Autodesk Inventor part; units mm, degrees
ref_plane "YZ Plane" through (0, 0, 0) normal (1, 0, 0) x (0, 1, 0)
ref_plane "XZ Plane" through (0, 0, 0) normal (0, 1, 0) x (-1, 0, 0)
ref_plane "XY Plane" through (0, 0, 0) normal (0, 0, 1) x (1, 0, 0)
sketch "Sketch1" plane through (0, 0, 0) normal (0, 0, 1) x (1, 0, 0)
  line L0 (-14.5, 28) -> (14.5, 28)
  line L1 (14.5, 28) -> (14.5, -28)
  line L2 (14.5, -28) -> (-14.5, -28)
  line L3 (-14.5, -28) -> (-14.5, 28)
  line L4 (17.5, 31) -> (-17.5, 31)
  line L5 (-17.5, 31) -> (-17.5, -31)
  line L6 (-17.5, -31) -> (17.5, -31)
  line L7 (14.5, -1.5) -> (26.5, -1.5)
  line L8 (14.5, -14.5) -> (26.5, -14.5)
  line L9 (17.5, -31) -> (17.5, -14.5)
  line L10 (17.5, -1.5) -> (17.5, 31)
  line L11 (26.5, -1.5) -> (26.5, -5)
  line L12 (26.5, -5) -> (14.5, -5)
  line L13 (26.5, -14.5) -> (26.5, -11)
  line L14 (26.5, -11) -> (14.5, -11)
  point P0 (0, 0)
  dimension "d0" = 29
  dimension "d1" = 56
  dimension "d2" = 14.5
  dimension "d3" = 28
  dimension "d4" = 3
  dimension "d5" = 12
  dimension "d6" = 3.5
  dimension "d7" = 3.5
  dimension "d8" = 6
  dimension "d9" = 32.5
  dimension "d10" = 62
extrude "Extrusion1" add sketch "Sketch1" along normal blind 10 contours L3 L2 L1 L8 L9 L6 L5 L4 L10 L7 L0 | L7 L11 L12 L1 | L1 L14 L13 L8
sketch "Sketch2" plane through (17.5, -1.5, 0) normal (0, 1, 0) x (1, 0, 0)
  line L0 (0, 0) -> (0, -10)
  line L1 (9, -10) -> (0, -10)
  line L2 (9, 0) -> (9, -10)
  line L3 (9, 0) -> (0, 0)
  point P0 (-17.5, 0)
  point P1 (5, -5)
  dimension "d13" = 4
hole "Hole1" at (22.5, -1.5, 5) direction (0, -1, 0) diameter 4 depth 13
chamfer "Chamfer1" distance 1 angle 45 4 edges at (26.5, -3.25, 0) (26.5, -3.25, 10) (26.5, -12.75, 10) (26.5, -12.75, 0)
fillet "Fillet1" radius 6 2 edges at (17.5, -14.5, 5) (17.5, -1.5, 5)
sketch "Sketch3" plane through (26.5, -1.5, 9) normal (0, 1, 0) x (1, 0, 0)
  line L0 (-3, -1) -> (-3, 2.2679)
  line L1 (-1, -1) -> (-3, -1)
  line L2 (0, 0) -> (-1, -1)
  line L3 (0, 8) -> (0, 0)
  line L4 (-1, 9) -> (0, 8)
  line L5 (-1, 9) -> (-3, 9)
  line L6 (-3, 5.7321) -> (-3, 9)
  arc A0 (-3, 2.2679) -> (-3, 5.7321) centre (-4, 4) ccw
  circle A1 centre (-4, 4) radius 4
  point P0 (-26.5, 9)
  dimension "d25" = 8
extrude "Extrusion2" cut sketch "Sketch3" along normal blind 10 contours A1 L6 A0 L0 | L0 A0 L6 A1
sketch "Sketch4" plane through (26.5, -14.5, 1) normal (0, -1, 0) x (1, 0, 0)
  line L0 (-3, -1) -> (-3, 2.2679)
  line L1 (-3, -1) -> (-1, -1)
  line L2 (0, 0) -> (-1, -1)
  line L3 (0, 0) -> (0, 8)
  line L4 (-1, 9) -> (0, 8)
  line L5 (-3, 9) -> (-1, 9)
  line L6 (-3, 5.7321) -> (-3, 9)
  arc A0 (-3, 2.2679) -> (-3, 5.7321) centre (-4, 4) ccw
  circle A1 centre (-4, 4) radius 4
  point P0 (-26.5, -1)
  dimension "d28" = 8
extrude "Extrusion3" cut sketch "Sketch4" along normal blind 10 contours A1 L6 A0 L0 | L0 A0 L6 A1
fillet "Fillet2" radius 3 4 edges at (17.5, 31, 5) (-17.5, 31, 5) (-17.5, -31, 5) (17.5, -31, 5)
equation "\"d7\" = d6"
properties part number "3DP_PLA_Battery_mount"
Can you work these out from the model? Positions are in its coordinate system, mm. A direction names the side the tool comes from. Round coordinates to 2 decimals unless told otherwise and drop trailing zeros. Order: outer loops, then holes, each group sorted by start corner. A loop starts at its lowest first (then second) coordinate and runs counter-clockwise, first axis right, second up. Notation, with made-up numbers: (11.25, 19.5) -> (22.25, 19.5) arc R21 cw to (22.25, 31.5) -> close; hole circle Ø6 at (24, 84). An arc over 180 degrees is marked (long way). Return JSON: item names as keys, results as strings. Group by question number.
1. If we section it at B-B, the plane z = 5: Count the separate pieces of the cut face and the enclosed holes in it, then the cut area to 3 significant figures.
2. If we section it at A-A, the plane y = 5.5: Write out the boundary of the cut face in (x, z).
3. If we section it at D-D, the plane x = 22.5: Write out the boundary of the cut face in (y, z).
4. We'd pull the mould along X, two halves only. Please class faces 4 (the face through (20.6, -11, 3.8)), 5 (the face through (-17.5, 0, 5)), 6 (the face through (14.5, -19, 5)), 7 (the face through (14.5, 12, 5)): released by +X, released by -X, zero draft, split by the parting line, or undercut.
5. Which directions (+Z, -Z, +X, -X, +Y, -Y) give clear straight access to the entire face, cutting with the end or side of a thin tool? Please do faces 1 (the face through (25, -14.5, 5)), 2 (the face through (-14.5, 0, 5)), 3 (the face through (16.6, 30.14, 4.93)).
6. If we section it at C-C, the plane x = -3.5: Write out the boundary of the cut face in (y, z).
7. I need wall thicknesses on line 1 (X direction, y = -12.2, z = 5); line 2 (Y direction, x = 6, z = 3.25); line 3 (X direction, y = -16.2, z = 5). Which ranges of each line are inside material? Lowest first, please. Write a range as [from, to].
8. Will these pins go through, and if not, where does the flat tip stop? pin 1 (5 mm diameter, centred on x = 22.5, z = 5, fed in from +Y); pin 2 (4 mm diameter, centred on y = -18.5, z = 4, fed in from +X); pin 3 (3 mm diameter, centred on x = 17, z = 8, fed in from +Y).
Output values:
{
 "1": {"separate pieces": "3", "enclosed holes": "0", "area": "563 mm²"},
 "2": {"outline": "(-17.5, 0) -> (-14.5, 0) -> (-14.5, 10) -> (-17.5, 10) -> close; (14.5, 0) -> (17.5, 0) -> (17.5, 10) -> (14.5, 10) -> close"},
 "3": {"outline": "(-14.58, 0) -> (-11, 0) -> (-11, 3) -> (-14.5, 3) -> (-14.5, 1) -> (-14.58, 1) -> close; (-14.58, 9) -> (-14.5, 9) -> (-14.5, 7) -> (-11, 7) -> (-11, 10) -> (-14.58, 10) -> close; (-5, 0) -> (-1.42, 0) -> (-1.42, 1) -> (-1.5, 1) -> (-1.5, 3) -> (-5, 3) -> close; (-5, 7) -> (-1.5, 7) -> (-1.5, 9) -> (-1.42, 9) -> (-1.42, 10) -> (-5, 10) -> close"},
 "4": {"face 4": "zero draft", "face 5": "released by -X", "face 6": "undercut", "face 7": "undercut"},
 "5": {"face 1": "+X, -Y", "face 2": "+Z, -Z", "face 3": "+Z, -Z, +X, +Y"},
 "6": {"outline": "(-31, 0) -> (-28, 0) -> (-28, 10) -> (-31, 10) -> close; (28, 0) -> (31, 0) -> (31, 10) -> (28, 10) -> close"},
 "7": {"line 1": "[-17.5, -14.5], [14.5, 20.5], [24.5, 26.5]", "line 2": "[-31, -28], [28, 31]", "line 3": "[-17.5, -14.5], [14.5, 18.5]"},
 "8": {"pin 1": "y = -1.5", "pin 2": "x = 18.9", "pin 3": "y = 30.83"}
}
